Geometry: final body of the model. Coordinates: model frame, mm. A direction names the side the tool comes from. Give positions to 0.01 mm unless a question says otherwise; leave off trailing zeros. Write each loop counter-clockwise with the first axis right and the second up, starting at its lowest first coordinate (ties: lowest second). Pieces come first, ordered by that corner, then holes. Notation, with made-up numbers: (69, 38.5) -> (95, 38.5) arc R32 cw to (95, 72.5) -> close; hole circle Ø4 at (-20.5, -40). An arc over 180 degrees is marked (long way). Answer as a JSON object with one key per item and string values. Group by question number.
(1) Set-up query: faces 1 (the face through (-44, 138, 2)), 2 (the face through (37.6, 122.5, 2)). Return all of +Z, -Z, +X, -X, +Y, -Y with unobstructed straight access to the full face (end or side cutting, diameter ignored); none if empty.
(2) Material intervals for probe 1 along X at (y, z) = (107, 0.5); probe 2 along X at (y, z) = (130, 1.8); probe 3 along Y at (x, z) = (-15, 0.8), sorted ascending.
(3) Section query D-D on x = -37.5. Output: boundary loops of the cut face in (y, z).
(4) Draft query along Y for faces 3 (the face through (1, 71, 4)), 4 (the face through (44, 138, 2)), 5 (the face through (-40, 95, 2)). Return one class per face: +Y half, -Y half, draft (parallel to the pull), parting line (faces both ways), or undercut.
(5) Section query A-A on y = 130. Output: boundary loops of the cut face in (x, z).
(6) Section query C-C on y = 107. Output: boundary loops of the cut face in (x, z).
(7) Section query B-B on x = -15. Output: boundary loops of the cut face in (y, z).
(8) Contact query for flat-ended pins moving along their axis: pin 1 Ø2.5 at (x, y) = (-22.26, 130) entering from -Z; pin 2 Ø1.5 at (y, z) = (29.5, 3.5) entering from -X; pin 3 Ø1 at (x, z) = (25, 1) entering from -Y. Output: stop coordinate, or through.
from build123d import *

# Parameters (mm, degrees)
F0_W     = 45
F0_H     = 140
F1_DEPTH = 4
F2_R     = 5
F3_SIZE  = 42.5
F5_D     = 3
F8_DEPTH = 60.96641
F11_D    = 3
F13_D    = 3


with BuildPart() as f1:
    # F0 (on Top) → F1 (new body)
    with BuildSketch(Plane.XY):
        with Locations((22.5, 70)):
            Rectangle(F0_W, F0_H)
    extrude(amount=F1_DEPTH)

    # F2
    f2_edges = [f1.edges().sort_by_distance(p)[0] for p in [
        (45, 140, 2),
    ]]
    fillet(f2_edges, radius=F2_R)

    # F3
    f3_edges = [f1.edges().sort_by_distance(p)[0] for p in [
        (45, 0, 2),
    ]]
    chamfer(f3_edges, length=F3_SIZE)

    # F5 (through all)
    with Locations(Plane.XY.offset(4)):
        with Locations((15, 107), (15, 83)):
            Hole(F5_D / 2)

    # F7 (on face) → F8 (cut)
    with BuildSketch(Plane.XY.offset(4)):
        with BuildLine():
            ThreePointArc((35, 70), (37.5, 67.5), (40, 70))
            Line((40, 70), (40, 120))
            ThreePointArc((40, 120), (37.5, 122.5), (35, 120))
            Line((35, 120), (35, 70))
        make_face()
    extrude(amount=-F8_DEPTH, mode=Mode.SUBTRACT)

    # F9: F1 across plane


with BuildPart() as f1_1:
    add(f1.part)
    add(f1.part.mirror(Plane.YZ))

    # F11 (through all)
    with Locations(Plane.XY.offset(4)):
        with Locations((-22.259496, 130), (22.740504, 130)):
            Hole(F11_D / 2)

    # F13 (through all)
    with Locations(Plane.XY.offset(4)):
        with Locations((-8.5621, 18.652199), (9.4379, 18.652199)):
            Hole(F13_D / 2)


solid = f1_1.part
Answer list:
{
 "1": {"face 1": "+Z, -Z, -X, +Y", "face 2": "+Z, -Z"},
 "2": {"probe 1": "-45 to -40, -35 to -16.5, -13.5 to 13.5, 16.5 to 35, 40 to 45", "probe 2": "-45 to -23.76, -20.76 to 21.24, 24.24 to 45", "probe 3": "12.5 to 81.5, 84.5 to 105.5, 108.5 to 140"},
 "3": {"outline": "(35, 0) -> (67.5, 0) -> (67.5, 4) -> (35, 4) -> close; (122.5, 0) -> (140, 0) -> (140, 4) -> (122.5, 4) -> close"},
 "4": {"face 3": "draft", "face 4": "+Y half", "face 5": "undercut"},
 "5": {"outline": "(-45, 0) -> (-23.76, 0) -> (-23.76, 4) -> (-45, 4) -> close; (-20.76, 0) -> (21.24, 0) -> (21.24, 4) -> (-20.76, 4) -> close; (24.24, 0) -> (45, 0) -> (45, 4) -> (24.24, 4) -> close"},
 "6": {"outline": "(-45, 0) -> (-40, 0) -> (-40, 4) -> (-45, 4) -> close; (-35, 0) -> (-16.5, 0) -> (-16.5, 4) -> (-35, 4) -> close; (-13.5, 0) -> (13.5, 0) -> (13.5, 4) -> (-13.5, 4) -> close; (16.5, 0) -> (35, 0) -> (35, 4) -> (16.5, 4) -> close; (40, 0) -> (45, 0) -> (45, 4) -> (40, 4) -> close"},
 "7": {"outline": "(12.5, 0) -> (81.5, 0) -> (81.5, 4) -> (12.5, 4) -> close; (84.5, 0) -> (105.5, 0) -> (105.5, 4) -> (84.5, 4) -> close; (108.5, 0) -> (140, 0) -> (140, 4) -> (108.5, 4) -> close"},
 "8": {"pin 1": "through", "pin 2": "x = -32.75", "pin 3": "y = 22"}
}
